Source: three-view drawing plus pictorial views. Frame: mm from the lowest corner of the part. A direction names the side the tool comes from. Give positions to 0.01 mm unless a question says otherwise; leave off trailing zeros. Order: outer loops, then holes, each group sorted by start corner. A loop starts at its lowest first (then second) coordinate and runs counter-clockwise, first axis right, second up.
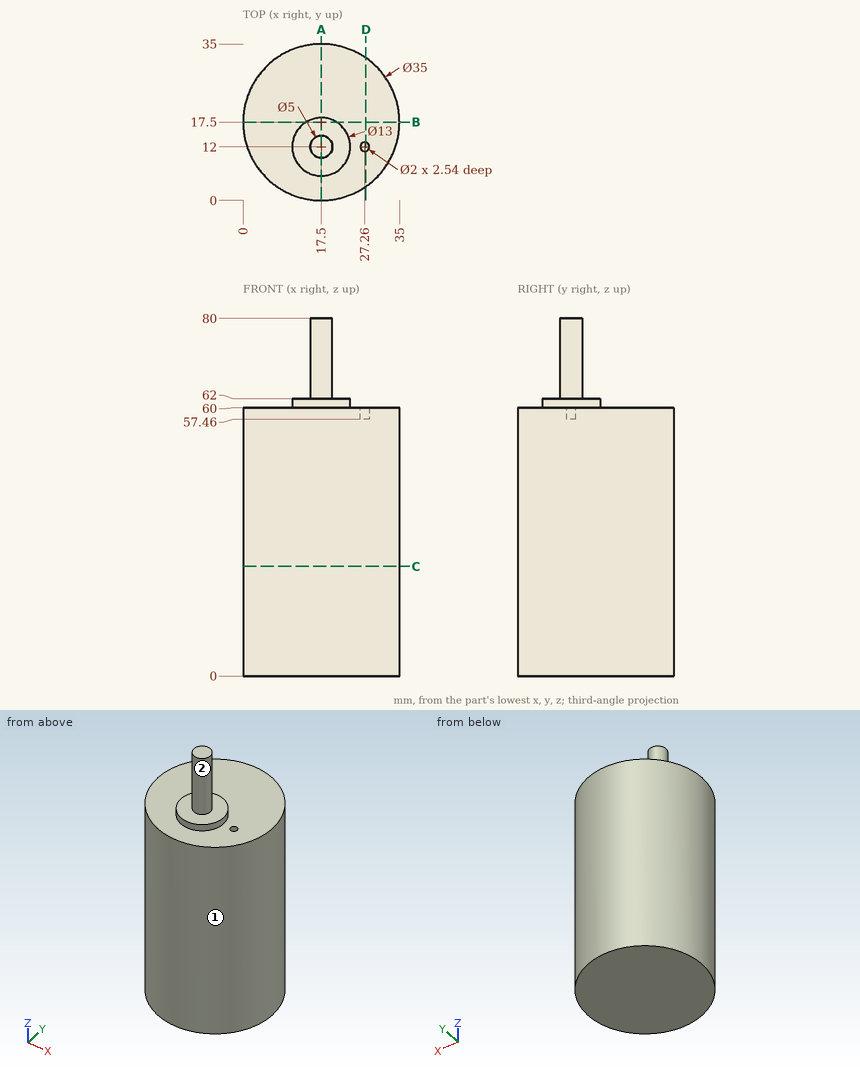
1) Section query A-A on x = 17.5. Output: boundary loops of the cut face in (y, z), and give its area (3 significant figures).
Checks:
outline: (0, 0) - (35, 0) - (35, 60) - (18.5, 60) - (18.5, 62) - (14.5, 62) - (14.5, 80) - (9.5, 80) - (9.5, 62) - (5.5, 62) - (5.5, 60) - (0, 60) - close
area: 2,220 mm2
2) Section query C-C on z = 24.5. Output: boundary loops of the cut face in (x, y), and give its area (3 significant figures).
Checks:
outline: circle Ø35 at (17.5, 17.5)
area: 962 mm2
3) First-contact query: pin 1 Ø1 at (x, y) = (5, 7.5) entering from +Z; pin 2 Ø8 at (x, z) = (5.5, 61) entering from -Y; pin 3 Ø10 at (x, y) = (8, 12.5) entering from +Z. Flat tips, straight axial feed; report the tip coordinate or a pass-through.
Checks:
pin 1: stops at z = 60
pin 2: stops at y = 2
pin 3: stops at z = 62
4) Section query D-D on x = 27.5. Output: boundary loops of the cut face in (y, z), and give its area (3 significant figures).
Checks:
outline: (3.14, 0) - (31.86, 0) - (31.86, 60) - (12.97, 60) - (12.97, 57.46) - (11.03, 57.46) - (11.03, 60) - (3.14, 60) - close
area: 1,720 mm2
5) Ray query, L1, parallel to Z at x = 9, y = 6; L2, parallel to Z at x = 20.5, y = 14.5; L3, parallel to Y at x = 17, z = 25.5. Return the intervals inside material, ascending.
Checks:
L1: z = 0 to 60
L2: z = 0 to 62
L3: y = 0.01 to 34.99
6) Section query B-B on y = 17.5. Output: boundary loops of the cut face in (x, z).
Checks:
outline: (0, 0) - (35, 0) - (35, 60) - (20.96, 60) - (20.96, 62) - (14.04, 62) - (14.04, 60) - (0, 60) - close
7) Reachability of the marked faces 1 and 2 from +Z, -Z, +X, -X, +Y, -Y: full face, straight path, thin tool, end or side. Return the list, or none.
Checks:
face 1: +Z, -Z
face 2: +Z
